Could you check a few things on this model? Use its own coordinates, in mm. Face numbers are marked on the shaded views. A direction names the side the tool comes from. Round coordinates to 2 decimals unless told otherwise and drop trailing zeros. Loops run counter-clockwise (first coordinate to the right, second up) from the corner with the lowest first, then second, coordinate; pieces in that order, holes last. Notation, with made-up numbers: (75, 55) -> (124, 55) arc R29 ccw to (124, 88) -> close; hole circle Ø6 at (82.25, -4). An arc over 180 degrees is marked (long way). One line per item, written item: value.
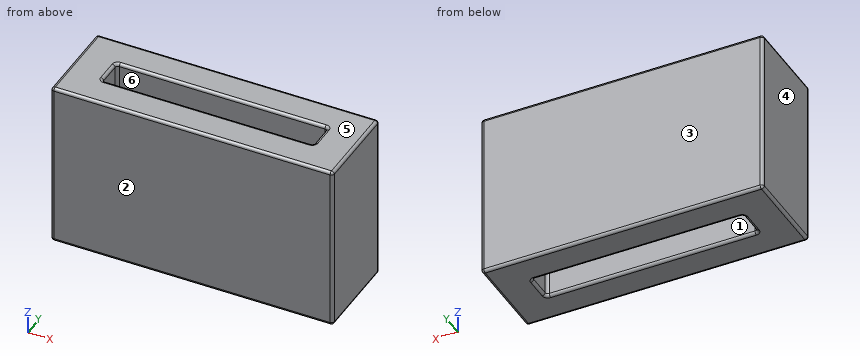
```python
from build123d import *

# Parameters (mm, degrees)
SKETCH1_W           = 100
SKETCH1_H           = 60
BOSS_EXTRUDE1_DEPTH = 32
SKETCH2_W           = 75
SKETCH2_H           = 10
CUT_EXTRUDE1_DEPTH  = 85.403791384
FILLET2_R           = 1


with BuildPart() as part:
    # Sketch1 → Boss-Extrude1 (new body)
    with BuildSketch(Plane(origin=(0, 0, 0), x_dir=(1, 0, 0), z_dir=(0, 1, 0))):
        Rectangle(SKETCH1_W, SKETCH1_H)
    extrude(amount=BOSS_EXTRUDE1_DEPTH)

    # Sketch2 → Cut-Extrude1 (cut, through all)
    with BuildSketch(Plane.XY.offset(30)):
        with Locations((0, 16)):
            Rectangle(SKETCH2_W, SKETCH2_H)
    extrude(amount=-CUT_EXTRUDE1_DEPTH, mode=Mode.SUBTRACT)

    # Fillet2
    fillet2_edges = [part.edges().sort_by_distance(p)[0] for p in [
        (-50, 32, 0),
        (0, 32, 30),
        (-37.5, 16, -30),
        (-37.5, 11, 0),
        (0, 21, -30),
        (-37.5, 21, 0),
        (37.5, 16, -30),
        (37.5, 21, 0),
        (0, 11, -30),
        (37.5, 11, 0),
        (-37.5, 16, 30),
        (0, 11, 30),
        (37.5, 16, 30),
        (0, 21, 30),
        (50, 32, 0),
        (0, 0, 30),
        (-50, 0, 0),
        (0, 0, -30),
        (50, 0, 0),
        (50, 16, 30),
        (-50, 16, 30),
        (-50, 16, -30),
        (50, 16, -30),
        (0, 32, -30),
    ]]
    fillet(fillet2_edges, radius=FILLET2_R)


solid = part.part
```
(1) Imagine slicing it at A-A on x = -1. Write out the boundary of the cut face in (y, z), then the cut area to 3 significant figures.
Results below:
outline: (0, -29) arc R1 ccw to (1, -30) -> (10, -30) arc R1 ccw to (11, -29) -> (11, 29) arc R1 ccw to (10, 30) -> (1, 30) arc R1 ccw to (0, 29) -> close; (21, -29) arc R1 ccw to (22, -30) -> (31, -30) arc R1 ccw to (32, -29) -> (32, 29) arc R1 ccw to (31, 30) -> (22, 30) arc R1 ccw to (21, 29) -> close
area: 1,320 mm²
(2) Imagine slicing it at B-B on y = 14.5. Write out the boundary of the cut face in (x, z), then the cut area to 3 significant figures.
Results below:
outline: (-50, -29) arc R1 ccw to (-49, -30) -> (-38.5, -30) arc R1 ccw to (-37.5, -29) -> (-37.5, 29) arc R1 ccw to (-38.5, 30) -> (-49, 30) arc R1 ccw to (-50, 29) -> close; (37.5, -29) arc R1 ccw to (38.5, -30) -> (49, -30) arc R1 ccw to (50, -29) -> (50, 29) arc R1 ccw to (49, 30) -> (38.5, 30) arc R1 ccw to (37.5, 29) -> close
area: 1,500 mm²
(3) Imagine slicing it at C-C on z = -7. Write out the boundary of the cut face in (x, y).
Results below:
outline: (-50, 1) arc R1 ccw to (-49, 0) -> (49, 0) arc R1 ccw to (50, 1) -> (50, 31) arc R1 ccw to (49, 32) -> (-49, 32) arc R1 ccw to (-50, 31) -> close; hole (-37.5, 12) arc R1 ccw to (-36.5, 11) -> (36.5, 11) arc R1 ccw to (37.5, 12) -> (37.5, 20) arc R1 ccw to (36.5, 21) -> (-36.5, 21) arc R1 ccw to (-37.5, 20) -> close
(4) We'd pull the mould along Y, two halves only. Please class the marked faces 1, 2, 3 and 4: +Y half, -Y half, draft (parallel to the pull), parting line (faces both ways), or undercut.
Results below:
face 1: undercut
face 2: -Y half
face 3: +Y half
face 4: draft
(5) Please list where these lines run through material, in increasing order: L1, parallel to X at y = 20, z = -19; L2, parallel to Y at x = -1, z = -19.5.
Results below:
L1: x = -50 to -37.5, 37.5 to 50
L2: y = 0 to 11, 21 to 32
(6) On a 3-axis mill with a long thin cutter (end or side, diameter ignored), from which of +Z, -Z, +X, -X, +Y, -Y can I reach the whole of each face in a straight line? I mean the marked faces 5 and 6. Say none if no direction works.
Results below:
face 5: +Z, +X, -X, +Y, -Y
face 6: +Z, -Z
